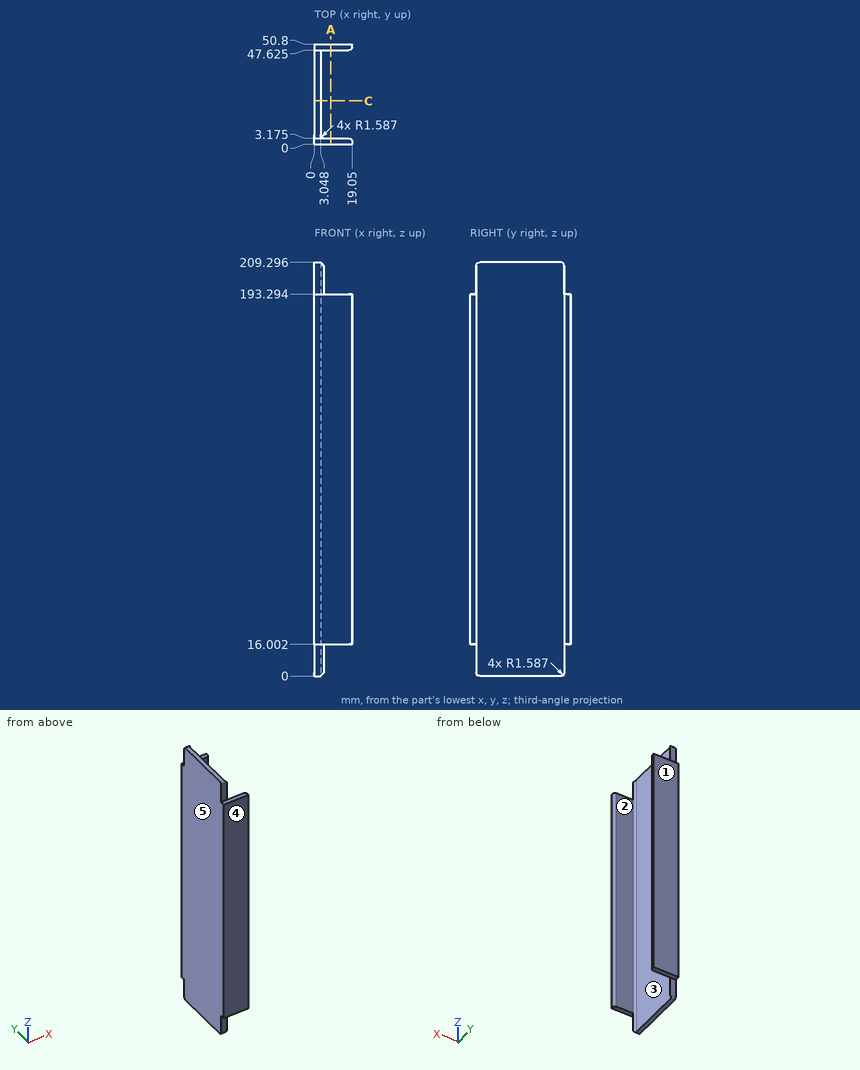
Source: three-view drawing plus pictorial views. Frame: mm from the lowest corner of the part. A direction names the side the tool comes from. Round coordinates to 2 decimals unless told otherwise and drop trailing zeros. Write each loop counter-clockwise with the first axis right and the second up, starting at its lowest first coordinate (ties: lowest second). Pieces come first, ordered by that corner, then holes. Notation, with made-up numbers: (61, -1.5) -> (79, -1.5) arc R25 ccw to (79, 30.5) -> close; hole circle Ø1 at (-27.5, 16.5). An arc over 180 degrees is marked (long way). Return JSON: item names as keys, results as strings.
Q1. First-contact query: pin 1 Ø1.6 at (x, y) = (14, 1) entering from +Z; pin 2 Ø1.4 at (x, z) = (2, 197) entering from +Y (1 decimal); pin 3 Ø2.5 at (x, z) = (2, 198.5) entering from -Y (1 decimal). Flat tips, straight axial feed; report the tip coordinate or a pass-through.
From the geometry:
{"pin 1": "z = 193.29", "pin 2": "y = 47.6", "pin 3": "y = 3.2"}
Q2. Section C-C on y = 22. Return the cut outline in (x, z) (1 decimal).
From the geometry:
{"outline": "(0, 0) -> (3, 0) -> (3, 209.3) -> (0, 209.3) -> close"}
Q3. Set-up query: the marked faces 1 and 2. Return all of +Z, -Z, +X, -X, +Y, -Y with unobstructed straight access to the full face (end or side cutting, diameter ignored); none if empty.
From the geometry:
{"face 1": "+Z, -Z, +X, -X, +Y", "face 2": "+Z, -Z, +X"}
Q4. Mould query, pull axis Y, two halves, no side actions, for the marked faces 3, 4 and 5. Classes: +Y half, -Y half, draft (parallel to the pull), parting line (faces both ways), or undercut.
From the geometry:
{"face 3": "undercut", "face 4": "-Y half", "face 5": "draft"}
Q5. Section A-A on x = 8.25. Return the cut outline in (y, z) (1 decimal), and give its area (3 significant figures).
From the geometry:
{"outline": "(0, 16) -> (3.2, 16) -> (3.2, 193.3) -> (0, 193.3) -> close; (47.6, 16) -> (50.8, 16) -> (50.8, 193.3) -> (47.6, 193.3) -> close", "area": "1,130 mm2"}
Q6. Ray query, line 1 (Y direction, x = 14.5, z = 148) (1 decimal); line 2 (Y direction, x = 17.75, z = 128.5); line 3 (X direction, y = 11, z = 27.5). Return the intervals inside material, ascending.
From the geometry:
{"line 1": "0 to 3.2, 47.6 to 50.8", "line 2": "0 to 3.15, 47.65 to 50.8", "line 3": "0 to 3.05"}
